from build123d import *

# Parameters (mm, degrees)
BOSS_EXTRUDE1_DEPTH  = 19.05
BOSS_EXTRUDE2_DEPTH  = 19.05
BOSS_EXTRUDE3_DEPTH  = 19.05
BOSS_EXTRUDE4_DEPTH  = 19.05
BOSS_EXTRUDE5_DEPTH  = 19.05
BOSS_EXTRUDE6_DEPTH  = 19.05
BOSS_EXTRUDE7_DEPTH  = 19.05
BOSS_EXTRUDE8_DEPTH  = 19.05
BOSS_EXTRUDE9_DEPTH  = 19.05
BOSS_EXTRUDE10_DEPTH = 19.05
BOSS_EXTRUDE11_DEPTH = 19.05
SKETCH12_W           = 38.1
SKETCH12_H           = 35.941255032
BOSS_EXTRUDE12_DEPTH = 19.05


with BuildPart() as part:
    # Sketch1 → Boss-Extrude1 (new body)
    with BuildSketch(Plane.XY):
        Polygon((0, 0), (114.3, 5.990209172), (133.35, 5.990209172), (133.35, 0), align=None)
    extrude(amount=BOSS_EXTRUDE1_DEPTH)

    # Sketch2 → Boss-Extrude2 (add)
    with BuildSketch(Plane(origin=(133.35, 0, 0), x_dir=(0, 0, -1), z_dir=(1, 0, 0))):
        Polygon((0, 0), (0, 5.990209172), (95.25, 10.982050149), (114.3, 10.982050149), (114.3, 0), align=None)
    extrude(amount=-BOSS_EXTRUDE2_DEPTH)

    # Sketch3 → Boss-Extrude3 (add)
    with BuildSketch(Plane(origin=(0, 0, -114.3), x_dir=(-1, 0, 0), z_dir=(0, 0, -1))):
        Polygon((-114.3, 0), (-114.3, 10.982050149), (-19.05, 15.973891125), (0, 15.973891125), (0, 0), align=None)
    extrude(amount=-BOSS_EXTRUDE3_DEPTH)

    # Sketch4 → Boss-Extrude4 (add)
    with BuildSketch(Plane.ZY):
        Polygon((-95.25, 15.973891125), (-19.05, 19.967363907), (0, 19.967363907), (0, 0), (-95.25, 0), align=None)
    extrude(amount=-BOSS_EXTRUDE4_DEPTH)

    # Sketch5 → Boss-Extrude5 (add)
    with BuildSketch(Plane.XY):
        Polygon((95.25, 23.960836688), (19.05, 19.967363907), (19.05, 0), (114.3, 0), (114.3, 23.960836688), align=None)
    extrude(amount=-BOSS_EXTRUDE5_DEPTH)

    # Sketch6 → Boss-Extrude6 (add)
    with BuildSketch(Plane(origin=(114.3, 0, 0), x_dir=(0, 0, -1), z_dir=(1, 0, 0))):
        Polygon((19.05, 23.960836688), (76.2, 26.955941274), (95.25, 26.955941274), (95.25, 0), (19.05, 0), align=None)
    extrude(amount=-BOSS_EXTRUDE6_DEPTH)

    # Sketch7 → Boss-Extrude7 (add)
    with BuildSketch(Plane(origin=(0, 0, -95.25), x_dir=(-1, 0, 0), z_dir=(0, 0, -1))):
        Polygon((-95.25, 26.955941274), (-38.1, 29.95104586), (-19.05, 29.95104586), (-19.05, 0), (-95.25, 0), align=None)
    extrude(amount=-BOSS_EXTRUDE7_DEPTH)

    # Sketch8 → Boss-Extrude8 (add)
    with BuildSketch(Plane.ZY.offset(-19.05)):
        Polygon((-76.2, 29.95104586), (-38.1, 31.947782251), (-19.05, 31.947782251), (-19.05, 0), (-76.2, 0), align=None)
    extrude(amount=-BOSS_EXTRUDE8_DEPTH)

    # Sketch9 → Boss-Extrude9 (add)
    with BuildSketch(Plane.XY.offset(-19.05)):
        Polygon((38.1, 31.947782251), (76.2, 33.944518642), (95.25, 33.944518642), (95.25, 0), (38.1, 0), align=None)
    extrude(amount=-BOSS_EXTRUDE9_DEPTH)

    # Sketch10 → Boss-Extrude10 (add)
    with BuildSketch(Plane(origin=(95.25, 0, 0), x_dir=(0, 0, -1), z_dir=(1, 0, 0))):
        Polygon((38.1, 0), (38.1, 33.944518642), (57.15, 34.942886837), (76.2, 34.942886837), (76.2, 0), align=None)
    extrude(amount=-BOSS_EXTRUDE10_DEPTH)

    # Sketch11 → Boss-Extrude11 (add)
    with BuildSketch(Plane(origin=(0, 0, -76.2), x_dir=(-1, 0, 0), z_dir=(0, 0, -1))):
        Polygon((-76.2, 34.942886837), (-57.15, 35.941255032), (-38.1, 35.941255032), (-38.1, 0), (-76.2, 0), align=None)
    extrude(amount=-BOSS_EXTRUDE11_DEPTH)

    # Sketch12 → Boss-Extrude12 (add)
    with BuildSketch(Plane.XY.offset(-57.15)):
        with Locations((57.15, 17.970627516)):
            Rectangle(SKETCH12_W, SKETCH12_H)
    extrude(amount=BOSS_EXTRUDE12_DEPTH)


solid = part.part
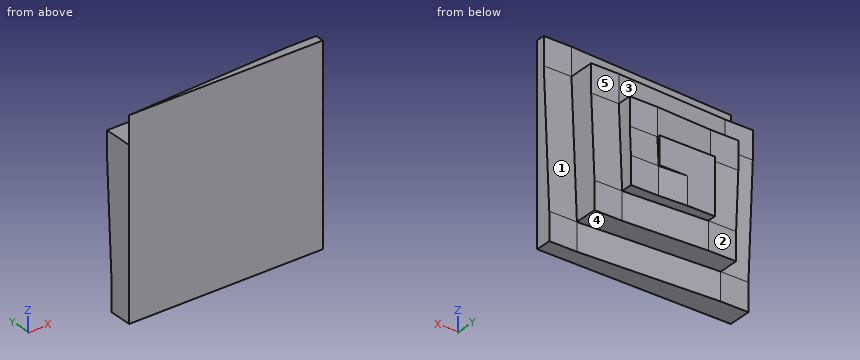
The listing builds one solid part. Answer for the finished solid, in the listing's coordinates (mm). Face numbers are marked on the shaded views. A direction names the side the tool comes from. Give positions to 0.01 mm unless a question says otherwise; leave off trailing zeros. Loops run counter-clockwise (first coordinate to the right, second up) from the corner with the lowest first, then second, coordinate; pieces in that order, holes last. Notation, with made-up numbers: (-34, 50.5) - (21, 50.5) arc R24 cw to (21, 82.5) - close; hole circle Ø11 at (63, 24.5). An arc over 180 degrees is marked (long way). Write each question's results on one line, items separated by ' | '.
1. Consider probe 1 along X at (y, z) = (13, -53); probe 2 along Z at (x, y) = (97, 17.5); probe 3 along Z at (x, y) = (40.5, 29.5). Determine where each line is inside the solid, lowest interval first. Write a range as from..to.
Resolved:
probe 1: x = 0..114.3 | probe 2: z = -95.25..0 | probe 3: z = -95.25..-19.05
2. Which of the six approach directions +Z, -Z, +X, -X, +Y, -Y give full straight-line access (tool end or side, diameter ignored) to the marked faces 1, 2, 3, 4 and 5?
Resolved:
face 1: +Z, +X, +Y | face 2: -Z, +X, -X, +Y | face 3: +Z, -X, +Y | face 4: -Z, +X, +Y | face 5: +Z, +X, -X, +Y
3. Find section D-D, the plane x = 116. Write down the section's boundary in (y, z).
Resolved:
outline: (0, -114.3) - (10.98, -114.3) - (10.98, -95.25) - (5.99, 0) - (5.99, 19.05) - (0, 19.05) - close
4. Find section A-A, the plane x = 98. Write down the section's boundary in (y, z), then the cut area to 3 significant figures.
Resolved:
outline: (0, -114.3) - (11.84, -114.3) - (11.84, -95.25) - (26.96, -95.25) - (26.96, -76.2) - (23.96, -19.05) - (23.96, 0) - (5.14, 0) - (5.14, 19.05) - (0, 19.05) - close | area: 2,750 mm^2
5. Find section C-C, the plane y = 8.5. Write down the section's boundary in (x, z).
Resolved:
outline: (0, -114.3) - (133.35, -114.3) - (133.35, -47.89) - (114.3, -47.89) - (114.3, 0) - (0, 0) - close
6. Flat-ended cylindrical pins translate along their axes: P1, Ø9.5, axis at x = 31.5, z = -33, coming from the +Y side; P2, Ø9.5, axis at x = 100, z = -10, coming from the +Y side; P3, Ø1.5, axis at y = 22.5, z = -4, coming from the +X side. Find the tip coordinate at first contact, or state that the pin passes through.
Resolved:
P1: stops at y = 31.95 | P2: stops at y = 23.96 | P3: stops at x = 114.3
7. Find section B-B, the plane z = -2.5. Write down the section's boundary in (x, y), then the cut area to 3 significant figures.
Resolved:
outline: (0, 0) - (133.35, 0) - (133.35, 6.12) - (114.3, 6.12) - (114.3, 23.96) - (95.25, 23.96) - (19.05, 19.97) - (0, 19.97) - close | area: 2,630 mm^2
